```python
from build123d import *

# Parameters (mm, degrees)
F0_R     = 50
F1_DEPTH = 570
F2_R     = 15
F3_DEPTH = 215
F4_R     = 15
F5_DEPTH = 245
F8_DEPTH = 4.5


with BuildPart() as f1:
    # F0 (on Right) → F1 (new body)
    with BuildSketch(Plane.YZ):
        Circle(F0_R)
    extrude(amount=F1_DEPTH)

    # F2 (on face) → F3 (join)
    with BuildSketch(Plane(origin=(0, 0, 0), x_dir=(0, -1, 0), z_dir=(-1, 0, 0))):
        Circle(F2_R)
    extrude(amount=F3_DEPTH)

    # F4 (on face) → F5 (join)
    with BuildSketch(Plane.YZ.offset(570)):
        Circle(F4_R)
    extrude(amount=F5_DEPTH)

    # F7 (on offset) → F8 (cut)
    with BuildSketch(Plane.XY.offset(15)):
        with BuildLine():
            ThreePointArc((810, 0), (808.828427, 2.828427), (806, 4))
            Line((806, 4), (782, 4))
            ThreePointArc((782, 4), (779.171573, 2.828427), (778, 0))
            ThreePointArc((778, 0), (779.171573, -2.828427), (782, -4))
            Line((782, -4), (806, -4))
            ThreePointArc((806, -4), (808.828427, -2.828427), (810, 0))
        make_face()
    extrude(amount=-F8_DEPTH, mode=Mode.SUBTRACT)


solid = f1.part
```
CAD build for the part. Positions are in the model's coordinates, mm. A direction names the side the tool comes from. Round coordinates to 2 decimals unless told otherwise and drop trailing zeros. Write each loop counter-clockwise with the first axis right and the second up, starting at its lowest first coordinate (ties: lowest second). Pieces come first, ordered by that corner, then holes. Notation, with made-up numbers: (-24.5, 0) - (5.5, 0) arc R20 cw to (5.5, 13) - close; hole circle Ø1 at (71, -33). An arc over 180 degrees is marked (long way). Write item = value, one per line. Start each with the question number.
Q1. Band-saw the part on D-D (x = 618). Give the cut face in (y, z), then the cut area to 3 significant figures.
Q2. Drop flat-ended pins along their axis: pin 1 (8 mm diameter, centred on y = 21, z = 38.5, fed in from +X); pin 2 (6 mm diameter, centred on x = 146.5, z = 7, fed in from -Y); pin 3 (2 mm diameter, centred on x = 370, z = -4, fed in from +Y). Give the stop position or say it passes through.
Q3. Band-saw the part on C-C (y = -35). Give the cut face in (x, z).
Q4. Probe L1, parallel to X at y = 27, z = -31; L2, parallel to Y at x = -108, z = 1.5; L3, parallel to Z at x = 90, y = 6. List the from-to ranges inside material, lowest first. Write a range as from..to.
Q5. Band-saw the part on A-A (z = 0). Give the cut face in (x, y), then the cut area to 3 significant figures.
Q6. Which spindle directions (+Z, -Z, +X, -X, +Y, -Y) get a long thin tool onto all of the face, cutting with end or side? Do faces 1 (the flat face through (570, -12, -10)), 2 (the flat face through (0, -12, -10)), 3 (the flat face through (815, 0, 0)). Say none if no direction does.
Q7. Band-saw the part on B-B (x = 237.5). Give the cut face in (y, z).
Answers below:
q1.outline = circle Ø30 at (0, 0)
q1.area = 707 mm2
q2.pin_1 = 570
q2.pin_2 = -49.84
q2.pin_3 = 49.91
q3.outline = (0, -35.71) - (570, -35.71) - (570, 35.71) - (0, 35.71) - close
q4.L1 = 0..570
q4.L2 = -14.92..14.92
q4.L3 = -49.64..49.64
q5.outline = (-215, -15) - (0, -15) - (0, -50) - (570, -50) - (570, -15) - (815, -15) - (815, 15) - (570, 15) - (570, 50) - (0, 50) - (0, 15) - (-215, 15) - close
q5.area = 70,800 mm2
q6.face_1 = +X
q6.face_2 = -X
q6.face_3 = +Z, -Z, +X, +Y, -Y
q7.outline = circle Ø100 at (0, 0)
